The model under review builds one solid part; all positions refer to its coordinate system, in mm. A direction names the side the tool comes from. Round coordinates to 2 decimals unless told otherwise and drop trailing zeros. Loops run counter-clockwise (first coordinate to the right, second up) from the corner with the lowest first, then second, coordinate; pieces in that order, holes last. Notation, with made-up numbers: (63.5, 27.5) - (112.5, 27.5) arc R20 ccw to (112.5, 39.5) - close; hole circle Ø4 at (59.5, 9.5). An arc over 180 degrees is marked (long way). Answer as CSV lines item,"result".
Autodesk Fusion 360 part; units mm, degrees
sketch "Sketch1" plane through (0, 0, 0) normal (0, 1, 0) x (1, 0, 0)
  line L0 (-26.25, -38.3437) -> (-55, -38.3437) construction
  arc A0 (18.3974, -42.2038) -> (34.374, -41.5937) centre (26.25, -38.3437) ccw
  arc A1 (45, -55) -> (55, -45) centre (45, -45) ccw
  line L1 (34.374, -41.5937) -> (35, -41.5937)
  arc A2 (0.8974, -42.2038) -> (-0.8974, -42.2038) centre (0, -42.6449) ccw
  arc A3 (18.3974, -42.2038) -> (16.6026, -42.2038) centre (17.5, -42.6449) ccw
  arc A4 (-34.374, -41.5937) -> (-18.3974, -42.2038) centre (-26.25, -38.3437) ccw
  arc A5 (-55, -45) -> (-45, -55) centre (-45, -45) ccw
  line L2 (-35, -29.5937) -> (35, -29.5937) construction
  line L3 (45, -45) -> (18.126, -41.5937) construction
  arc A6 (0.8974, -42.2038) -> (16.6026, -42.2038) centre (8.75, -38.3437) ccw
  line L4 (45, -55) -> (-45, -55)
  line L5 (-34.374, -41.5937) -> (-45, -45) construction
  line L6 (26.25, -38.3437) -> (55, -38.3437) construction
  arc A7 (-45, -31.5937) -> (-35, -41.5937) centre (-35, -31.5937) ccw
  line L7 (0, 0) -> (0, -57.946) construction
  arc A8 (-16.6026, -42.2038) -> (-18.3974, -42.2038) centre (-17.5, -42.6449) ccw
  arc A9 (-16.6026, -42.2038) -> (-0.8974, -42.2038) centre (-8.75, -38.3437) ccw
  arc A10 (35, -41.5937) -> (45, -31.5937) centre (35, -31.5937) ccw
  line L8 (-35, -41.5937) -> (-34.374, -41.5937)
  line L9 (-55, -45) -> (-55, 0)
  line L10 (-55, 0) -> (-45, 0)
  line L11 (-45, 0) -> (-45, -31.5937)
  line L12 (55, -45) -> (55, 0)
  line L13 (55, 0) -> (45, 0)
  line L14 (45, 0) -> (45, -31.5937)
  line L15 (55, 0) -> (-55, 0) construction
  dimension "d1" = 10
  dimension "d2" = 10
  dimension "d3" = 10
  dimension "d4" = 17.5
  dimension "d5" = 17.5
  dimension "d6" = 17.5
  dimension "d7" = 17.5
  dimension "d8" = 17.5
  dimension "d9" = 17.5
  dimension "d10" = 17.5
  dimension "d11" = 12
  dimension "d12" = 1
  dimension "d13" = 1
  dimension "d14" = 1
extrude "Extrude1" add sketch "Sketch1" along normal mid plane 20
fillet "Fillet1" radius 1 14 edges at (-26.5838, -10, 47.0874) (-17.5, -10, 41.6449) (-8.75, -10, 47.0937) (0, -10, 41.6449) (8.75, -10, 47.0937) (17.5, -10, 41.6449) (26.5838, -10, 47.0874) (26.5838, 10, 47.0874) (17.5, 10, 41.6449) (8.75, 10, 47.0937) (0, 10, 41.6449) (-8.75, 10, 47.0937) (-17.5, 10, 41.6449) (-26.5838, 10, 47.0874)
sketch "Sketch2" plane through (0, 0, 0) normal (0, 0, 1) x (1, 0, 0)
  circle A0 centre (-50, -5) radius 4
  circle A1 centre (-50, 5) radius 4
  circle A2 centre (50, -5) radius 4
  circle A3 centre (50, 5) radius 4
  dimension "d18" = 8
  dimension "d19" = 8
  dimension "d20" = 8
  dimension "d21" = 8
extrude "Extrude2" add sketch "Sketch2" against normal blind 10
1. Take a section at B-B (y = -5). State the section outline as (x, z) points, plus the area to 3 significant figures.
Numbers:
outline,"(-55, 0) - (-54, 0) - (-54, -10) - (-46, -10) - (-46, 0) - (-45, 0) - (-45, 31.59) arc R10 cw to (-35, 41.59) - (-34.37, 41.59) arc R8.75 cw to (-18.4, 42.2) arc R1 ccw to (-16.6, 42.2) arc R8.75 cw to (-0.9, 42.2) arc R1 ccw to (0.9, 42.2) arc R8.75 cw to (16.6, 42.2) arc R1 ccw to (18.4, 42.2) arc R8.75 cw to (34.37, 41.59) - (35, 41.59) arc R10 cw to (45, 31.59) - (45, 0) - (46, 0) - (46, -10) - (54, -10) - (54, 0) - (55, 0) - (55, 45) arc R10 ccw to (45, 55) - (-45, 55) arc R10 ccw to (-55, 45) - close"
area,"2,210 mm²"
2. Take a section at D-D (z = 39.5). State the section outline as (x, y) points.
Numbers:
outline,"(-55, -10) - (-41.12, -10) - (-41.12, 10) - (-55, 10) - close; (41.12, -10) - (55, -10) - (55, 10) - (41.12, 10) - close"
3. Draft analysis for pull direction X (two halves, no side actions). For faces 1 (the face through (-51.99, -0.14, 52.15)), 2 (the face through (50, 5, -10)), 3 (the face through (46, -5, -5)), 4 (the face through (52.15, -0.14, 51.99)), state which applies: +X half, -X half, draft (parallel to the pull), parting line (faces both ways), or undercut.
Numbers:
face 1,"-X half"
face 2,"draft"
face 3,"undercut"
face 4,"+X half"
4. Tool access review of faces 5 (the face through (0, 10, 44)), 6 (the face through (45, 0, 16)), 7 (the face through (46.8, 2.6, -4.9)): name each direction out of +Z, -Z, +X, -X, +Y, -Y from which nothing blocks a thin tool from reaching the whole face with its end or side.
Numbers:
face 5,"+Z, -Z, +X, -X, +Y"
face 6,"-Z, +Y, -Y"
face 7,"-Z"
5. Take a section at A-A (z = 3). State the section outline as (x, y) points, plus the area to 3 significant figures.
Numbers:
outline,"(-55, -10) - (-45, -10) - (-45, 10) - (-55, 10) - close; (45, -10) - (55, -10) - (55, 10) - (45, 10) - close"
area,"400 mm²"
6. Clearance check with flat-ended pins moving along their axes: pin 1 (0.7 mm diameter, centred on x = -34.5, y = 3.5, fed in from -Z); pin 2 (1.5 mm diameter, centred on x = -5.5, y = -0.5, fed in from -Z). State where each tip first meets the part, or that it passes through.
Numbers:
pin 1,"stops at z = 41.59"
pin 2,"stops at z = 46.13"
7. Take a section at C-C (x = 50). State the section outline as (y, z) points, plus the area to 3 significant figures.
Numbers:
outline,"(-10, 0) - (-9, 0) - (-9, -10) - (-1, -10) - (-1, 0) - (1, 0) - (1, -10) - (9, -10) - (9, 0) - (10, 0) - (10, 53.66) - (-10, 53.66) - close"
area,"1,230 mm²"
8. Wall thickness on probe 1 along X at (y, z) = (7.25, 4.5); probe 2 along X at (y, z) = (0.25, 46); probe 3 along X at (y, z) = (0.25, 34): over which ranges is each line inside the solid? List them lowest first.
Numbers:
probe 1,"x = -55 to -45, 45 to 55"
probe 2,"x = -54.95 to -30.49, -22.01 to -12.99, -4.51 to 4.51, 12.99 to 22.01, 30.49 to 54.95"
probe 3,"x = -55 to -44.71, 44.71 to 55"
